Autodesk Inventor part; units mm, degrees
ref_plane "YZ Plane" through (0, 0, 0) normal (1, 0, 0) x (0, 1, 0)
ref_plane "XZ Plane" through (0, 0, 0) normal (0, 1, 0) x (-1, 0, 0)
ref_plane "XY Plane" through (0, 0, 0) normal (0, 0, 1) x (1, 0, 0)
sketch "Sketch1" plane through (0, 0, 0) normal (0, 0, 1) x (1, 0, 0)
  line L0 (0, -9.713) -> (25.4, -9.713)
  line L1 (25.4, -9.713) -> (25.4, 9.337)
  line L2 (0, 9.337) -> (0, -9.713)
  line L3 (19.05, 9.337) -> (19.05, 15.687)
  line L4 (19.05, 15.687) -> (22.225, 15.687)
  line L5 (22.225, 15.687) -> (22.225, 9.337)
  line L6 (25.4, 9.337) -> (22.225, 9.337)
  line L7 (19.05, 9.337) -> (0, 9.337)
  dimension "d0" = 19.05
  dimension "d2" = 25.4
  dimension "d3" = 3.175
  dimension "d4" = 6.35
  dimension "d22" = 3.175
extrude "Extrusion1" add sketch "Sketch1" against normal blind 3.175
sketch "Sketch2" plane through (0, 0, 0) normal (0, 0, 1) x (1, 0, 0)
  line L0 (12.7, -1.7755) -> (19.05, -1.7755)
  line L1 (19.05, -1.7755) -> (19.05, 1.3995)
  line L2 (19.05, 1.3995) -> (12.7, 1.3995)
  line L3 (12.7, 1.3995) -> (12.7, -1.7755)
  line L4 (0, 9.337) -> (0, -9.713)
  line L5 (25.4, 9.337) -> (22.225, 9.337)
  line L6 (25.4, -9.713) -> (25.4, 9.337)
  dimension "d7" = 3.175
  dimension "d10" = 6.35
  dimension "d11" = 7.9375
  dimension "d12" = 6.35
extrude "Extrusion2" add sketch "Sketch2" along normal blind 12.7
sketch "Sketch3" plane through (22.225, 9.337, 0) normal (1, 0, 0) x (0, 0, -1)
  line L0 (0, 0) -> (0, 6.35)
  line L1 (0, 0) -> (3.175, 0)
  line L2 (3.175, 6.35) -> (3.175, 0)
  line L3 (0, 6.35) -> (3.175, 6.35)
  point P0 (1.5537, 4.7498)
  dimension "d38" = 1.6002
hole "Hole1" at (22.225, 14.0868, -1.5537) direction (-1, 0, 0) diameter 1.524 end through all
sketch "Sketch5" plane through (0, 0, -3.175) normal (0, 0, -1) x (-1, 0, 0)
  line L0 (-25.4, -9.713) -> (0, -9.713)
  line L1 (0, -9.713) -> (0, 9.337)
  line L2 (0, 9.337) -> (-19.05, 9.337)
  line L3 (-19.05, 9.337) -> (-19.05, 15.687)
  line L4 (-19.05, 15.687) -> (-22.225, 15.687)
  line L5 (-22.225, 15.687) -> (-22.225, 9.337)
  line L6 (-22.225, 9.337) -> (-25.4, 9.337)
  line L7 (-25.4, 9.337) -> (-25.4, -9.713)
  point P0 (-22.225, -11.491)
  point P1 (-4.8639, -0.1739)
  dimension "d37" = 3.175
hole "Hole3" at (4.8639, -0.1739, -3.175) at (22.225, -11.491, -3.175) direction (0, 0, 1) diameter 3.302 end through all
sketch "Sketch6" plane through (22.225, 9.337, 0) normal (1, 0, 0) x (0, 0, -1)
  point P0 (0, -9.337)
sketch "Sketch7" plane through (0, 0, 0) normal (0, 0, 1) x (1, 0, 0)
  point P0 (0, 0)
sketch "Sketch8" plane through (0, -9.713, 0) normal (0, -1, 0) x (1, 0, 0)
  line L0 (25.4, 0) -> (22.225, 0)
  line L1 (22.225, 0) -> (22.225, -3.175)
  line L2 (19.05, -3.175) -> (22.225, -3.175)
  line L3 (0, 0) -> (25.4, 0)
  line L4 (22.225, -3.175) -> (25.4, -3.175)
  line L5 (22.225, -3.175) -> (19.05, -3.175)
  line L6 (19.05, -3.175) -> (19.05, 0)
  line L7 (19.05, 0) -> (22.225, 0)
  line L8 (22.225, 0) -> (22.225, -3.175)
extrude "Extrusion3" add sketch "Sketch8" along normal blind 6.35
hole "Hole4" at (19.05, -14.4755, -1.5875) direction (1, 0, 0) diameter 1.524 depth 25.4 tip angle 118
hole "Hole5" at (15.875, -1.7755, 9.525) direction (0, 1, 0) diameter 3.175 depth 25.4 tip angle 118
equation "\"d11\" = -0.5 * d7 + 0.5 * d0"
properties part number "slide pivot plate"
Design review of the part built by this model. Coordinates are the model's own, in mm. A direction names the side the tool comes from. Coordinates: 2 decimals unless noted, no trailing zeros. Loops run counter-clockwise (first coordinate to the right, second up) from the corner with the lowest first, then second, coordinate; pieces in that order, holes last. Notation, with made-up numbers: (58.25, 64) -> (94.25, 64) arc R13 cw to (94.25, 74) -> close; hole circle Ø7 at (-23.75, -27). An arc over 180 degrees is marked (long way). Use a Markdown table: item, result. Add a question column.
Item 1: The part is to be moulded in two halves that separate along Y. For faces 1 (the flat face through (16, -1.776, 6)), 2 (the cylindrical face through (20.66, -14.184, -0.884)), 3 (the flat face through (19.05, -13, -2)), say which applies: +Y half, -Y half, draft (parallel to the pull), parting line (faces both ways), or undercut.
Item 2: Clearance check with flat-ended pins moving along their axes: P1, Ø2.5, axis at y = -14, z = -2, coming from the -X side; P2, Ø3, axis at x = 13.5, y = 10, coming from the +Z side; P3, Ø2, axis at x = 15.5, z = 0.5, coming from the +Y side; P4, Ø8, axis at y = -12.5, z = 7, coming from the -X side. State where each tip first meets the part, or that it passes through.
Item 3: Machinability: for faces 4 (the flat face through (16, 1.4, 6)), 5 (the flat face through (22.225, -13, -2)), 6 (the flat face through (22.225, 13, -2)), 7 (the flat face through (19.05, 0, 6)), which of the approach directions +Z, -Z, +X, -X, +Y, -Y give a long, thin tool a straight path to every point of the face, cutting with its end or side? Answer none if there is none.
Item 4: We need section C-C, the plane z = 10. Write out the cut boundary in (x, y), and give its area (3 significant figures).
Item 5: We need section D-D, the plane x = 19.5. Write out the cut boundary in (y, z) (1 decimal), and give its area (3 significant figures).
Item 6: We need section A-A, the plane z = -1.25. Write out the cut boundary in (x, y) (3 decimals).
Item 7: Wall thickness on L1, parallel to Z at x = 15.75, y = 3.5 (3 decimals); L2, parallel to Y at x = 14, z = 3; L3, parallel to X at y = 13.5, z = -0.75 (3 decimals): over which ranges is each line inside the solid? List them lowest first. Write a range as from..to.
Item 8: We need section B-B, the plane y = 5.5. Write out the cut boundary in (x, z) (3 decimals).
Numbers:
| question | item | result |
|---|---|---|
| 1 | face 1 | -Y half |
| 1 | face 2 | undercut |
| 1 | face 3 | draft |
| 2 | P1 | stops at x = 19.05 |
| 2 | P2 | stops at z = 0 |
| 2 | P3 | stops at y = 9.34 |
| 2 | P4 | passes through |
| 3 | face 4 | +Z, +X, -X, +Y |
| 3 | face 5 | +Z, -Z, +X, -Y |
| 3 | face 6 | +Z, -Z, +X, +Y |
| 3 | face 7 | +Z, +X, +Y, -Y |
| 4 | outline | (12.7, -1.78) -> (14.36, -1.78) -> (14.36, 1.4) -> (12.7, 1.4) -> close; (17.39, -1.78) -> (19.05, -1.78) -> (19.05, 1.4) -> (17.39, 1.4) -> close |
| 4 | area | 10.5 mm^2 |
| 5 | outline | (-16.1, -3.2) -> (15.7, -3.2) -> (15.7, 0) -> (-16.1, 0) -> close; hole circle Ø1.5 at (-14.5, -1.6); hole circle Ø1.5 at (14.1, -1.6) |
| 5 | area | 97.2 mm^2 |
| 6 | outline | (0, -9.713) -> (19.05, -9.713) -> (19.05, -13.792) -> (22.225, -13.792) -> (22.225, -9.713) -> (25.4, -9.713) -> (25.4, 9.337) -> (22.225, 9.337) -> (22.225, 13.388) -> (19.05, 13.388) -> (19.05, 9.337) -> (0, 9.337) -> close; (19.05, -16.063) -> (22.225, -16.063) -> (22.225, -15.159) -> (19.05, -15.159) -> close; (19.05, 14.786) -> (22.225, 14.786) -> (22.225, 15.687) -> (19.05, 15.687) -> close; hole circle Ø3.302 at (4.864, -0.174) |
| 7 | L1 | z = -3.175..0 |
| 7 | L2 | y = -1.78..1.4 |
| 7 | L3 | x = 19.05..22.225 |
| 8 | outline | (0, -3.175) -> (25.4, -3.175) -> (25.4, 0) -> (0, 0) -> close |
